Verification items for the finished model (mm, model axes). A direction names the side the tool comes from. Round coordinates to 2 decimals unless told otherwise and drop trailing zeros. Write each loop counter-clockwise with the first axis right and the second up, starting at its lowest first coordinate (ties: lowest second). Pieces come first, ordered by that corner, then holes. Notation, with made-up numbers: (-21, 4) - (33, 4) arc R19 ccw to (33, 28) - close; hole circle Ø7 at (43, -5). An arc over 180 degrees is marked (long way). Write each question's results on one line, items separated by ' | '.
```python
from build123d import *

# Parameters (mm, degrees)
SKETCH1_W           = 40
SKETCH1_H           = 19
BOSS_EXTRUDE1_DEPTH = 4
CUT_EXTRUDE1_REACH  = 24.5
SKETCH2_R           = 2.75
SKETCH4_W           = 16.5
SKETCH4_H           = 19
CUT_EXTRUDE2_DEPTH  = 1.5
FILLET1_R           = 5


with BuildPart() as part:
    # Sketch1 → Boss-Extrude1 (new body)
    with BuildSketch(Plane(origin=(0, 0, 0), x_dir=(1, 0, 0), z_dir=(0, 1, 0))):
        Rectangle(SKETCH1_W, SKETCH1_H)
    extrude(amount=BOSS_EXTRUDE1_DEPTH)

    # Sketch2 → Cut-Extrude1 (cut, up to next)
    with BuildSketch(Plane(origin=(0, 4, 0), x_dir=(1, 0, 0), z_dir=(0, 1, 0)), mode=Mode.PRIVATE) as cut_extrude1_sk1:
        with Locations(Location((10, 0, 0), (0, 0, 270))):
            Circle(SKETCH2_R)
    cut_extrude1_tool1 = extrude(cut_extrude1_sk1.sketch, amount=-CUT_EXTRUDE1_REACH, mode=Mode.PRIVATE) & part.part
    add(cut_extrude1_tool1.solids().sort_by_distance((10, 4, 0))[0], mode=Mode.SUBTRACT)

    # Sketch4 → Cut-Extrude2 (cut)
    with BuildSketch(Plane(origin=(0, 4, 0), x_dir=(1, 0, 0), z_dir=(0, 1, 0))):
        with Locations((-11.75, 0)):
            Rectangle(SKETCH4_W, SKETCH4_H)
        with BuildLine():
            Line((-7.9, 5), (-7.9, 2))
            ThreePointArc((-7.9, 2), (-9.3, 0.6), (-10.7, 2))
            Line((-10.7, 2), (-10.7, 5))
            ThreePointArc((-10.7, 5), (-9.3, 6.4), (-7.9, 5))
        make_face(mode=Mode.SUBTRACT)
        with BuildLine():
            Line((-12.1, -2), (-12.1, -5))
            ThreePointArc((-12.1, -5), (-13.5, -6.4), (-14.9, -5))
            Line((-14.9, -5), (-14.9, -2))
            ThreePointArc((-14.9, -2), (-13.5, -0.6), (-12.1, -2))
        make_face(mode=Mode.SUBTRACT)
    extrude(amount=-CUT_EXTRUDE2_DEPTH, mode=Mode.SUBTRACT)

    # Fillet1
    fillet1_edges = [part.edges().sort_by_distance(p)[0] for p in [
        (20, 2, 9.5),
        (20, 2, -9.5),
    ]]
    fillet(fillet1_edges, radius=FILLET1_R)


solid = part.part
```
(1) Section check D-D (z = -3.25). Record the cut outline in (x, y), plus the area to 3 significant figures.
Answer:
outline: (-20, 0) - (20, 0) - (20, 4) - (-3.5, 4) - (-3.5, 2.5) - (-7.9, 2.5) - (-7.9, 4) - (-10.7, 4) - (-10.7, 2.5) - (-20, 2.5) - close | area: 139 mm2
(2) Set-up check for faces 5 (the flat face through (-3.5, 3, 0)), 6 (the flat face through (-14.9, 3, 4)), 7 (the cylindrical face through (-9.3, 3.3, -0.6)): record each of +Z, -Z, +X, -X, +Y, -Y from which the full face is reachable in a straight line by a thin tool's end or side.
Answer:
face 5: +Z, -Z, +Y | face 6: +Z, -Z, -X, +Y | face 7: +Z, +Y
(3) Section check A-A (y = 3.55). Record the cut outline in (x, z), plus the area to 3 significant figures.
Answer:
outline: (-14.9, 2) arc R1.4 ccw to (-12.1, 2) - (-12.1, 5) arc R1.4 ccw to (-14.9, 5) - close; (-10.7, -5) arc R1.4 ccw to (-7.9, -5) - (-7.9, -2) arc R1.4 ccw to (-10.7, -2) - close; (-3.5, -9.5) - (15, -9.5) arc R5 ccw to (20, -4.5) - (20, 4.5) arc R5 ccw to (15, 9.5) - (-3.5, 9.5) - close; hole circle Ø5.5 at (10, 0) | area: 441 mm2
(4) Mould release check, pull along X, two halves, no side actions. Record for faces 1 (the flat face through (-7.9, 3, -4)), 2 (the flat face through (-12, 2.5, 0)), 3 (the flat face through (-20, 1, 0)), 4 (the cylindrical face through (18.5, 2.03, -8.07)): released by +X, released by -X, zero draft, split by the parting line, or undercut.
Answer:
face 1: undercut | face 2: undercut | face 3: released by -X | face 4: released by +X
(5) Thickness scan on L1, parallel to X at y = 3.7, z = -4; L2, parallel to X at y = 1, z = 0; L3, parallel to Y at x = -18, z = -2.5. Record the ranges inside material, lowest first.
Answer:
L1: -10.7 to -7.9, -3.5 to 20 | L2: -20 to 7.25, 12.75 to 20 | L3: 0 to 2.5
(6) Section check C-C (x = -9). Record the cut outline in (y, z).
Answer:
outline: (0, -9.5) - (2.5, -9.5) - (2.5, -6.37) - (4, -6.37) - (4, -0.63) - (2.5, -0.63) - (2.5, 9.5) - (0, 9.5) - close
(7) Section check B-B (z = 0). Record the cut outline in (x, y), plus the area to 3 significant figures.
Answer:
outline: (-20, 0) - (7.25, 0) - (7.25, 4) - (-3.5, 4) - (-3.5, 2.5) - (-20, 2.5) - close; (12.75, 0) - (20, 0) - (20, 4) - (12.75, 4) - close | area: 113 mm2
(8) Go/stop test with flat-tipped pins: pin 1 Ø1.2 at (y, z) = (3.5, 4) entering from -X; pin 2 Ø4 at (x, z) = (-4, -2) entering from +Y. Record where each tip stops, or that it passes through.
Answer:
pin 1: x = -14.9 | pin 2: y = 4
